from build123d import *

# Parameters (mm, degrees)
F0_W     = 115
F0_H     = 75
F1_DEPTH = 70
F2_W     = 60
F2_H     = 25
F3_DEPTH = 70
F4_W     = 10
F4_H     = 30
F5_DEPTH = 75
F6_W     = 30
F6_H     = 5
F6_W_2   = 15
F6_H_2   = 20
F7_DEPTH = 50
F8_W     = 25
F8_H     = 20
F9_DEPTH = 75


with BuildPart() as f1:
    # F0 (on Front) → F1 (new body)
    with BuildSketch(Plane.XZ):
        with Locations((57.5, 37.5)):
            Rectangle(F0_W, F0_H)
    extrude(amount=F1_DEPTH)

    # F2 (on face) → F3 (cut)
    with BuildSketch(Plane.XZ.offset(70)):
        with Locations((55, 62.5)):
            Rectangle(F2_W, F2_H)
    extrude(amount=-F3_DEPTH, mode=Mode.SUBTRACT)

    # F4 (on face) → F5 (cut)
    with BuildSketch(Plane.XY.offset(75)):
        with Locations((90, -55)):
            Rectangle(F4_W, F4_H)
    extrude(amount=-F5_DEPTH, mode=Mode.SUBTRACT)

    # F6 (on face) → F7 (cut)
    with BuildSketch(Plane.XY.offset(50)):
        Polygon((85, -70), (85, -40), (70, -40), (40, -40), (40, -50), (40, -70), align=None)
        with Locations((55, -37.5)):
            Rectangle(F6_W, F6_H)
        with Locations((32.5, -60)):
            Rectangle(F6_W_2, F6_H_2)
    extrude(amount=-F7_DEPTH, mode=Mode.SUBTRACT)

    # F8 (on face) → F9 (cut)
    with BuildSketch(Plane.XY.offset(75)):
        with Locations((12.5, -60)):
            Rectangle(F8_W, F8_H)
    extrude(amount=-F9_DEPTH, mode=Mode.SUBTRACT)


solid = f1.part
Design review of the part built by this model. Coordinates are the model's own, in mm. A direction names the side the tool comes from. Coordinates: 2 decimals unless noted, no trailing zeros. Order: outer loops, then holes, each group sorted by start corner. A loop starts at its lowest first (then second) coordinate and runs counter-clockwise, first axis right, second up. Notation, with made-up numbers: (-14, 85.25) -> (17, 85.25) arc R20 cw to (17, 117.25) -> close; hole circle Ø7 at (-10.5, 72.25). An arc over 180 degrees is marked (long way). Use one line per item in the form item = value. Start each with the question number.
(1) The part is to be moulded in two halves that separate along X. For faces 4 (the flat face through (0, -25, 37)), 5 (the flat face through (85, -20, 62)), 6 (the flat face through (115, -35, 37)), 7 (the flat face through (103, -35, 75)), say which applies: +X half, -X half, draft (parallel to the pull), parting line (faces both ways), or undercut.
(2) For faces 1 (the flat face through (20, -50, 38)), 2 (the flat face through (70, -38, 25)), 3 (the flat face through (25, -25, 63)), list the 3-axis set-ups (+Z, -Z, +X, -X, +Y, -Y) from which the entire face can be reached by the end or side of a thin tool; tool diameter is ignored.
(3) Add section D-D on x = 75.5. State the section outline as (y, z) points.
(4) Insertion check: pin 1 (3 mm diameter, centred on x = 63, y = -27, fed in from +Z); pin 2 (2 mm diameter, centred on x = 91, z = 23, fed in from -Y). Each pin has a flat end and moves straight along its axis. Give the tip position at first contact, or say it passes through.
(5) For probe 1 along X at (y, z) = (-36, 4.5); probe 2 along X at (y, z) = (-11, 64); probe 3 along Y at (x, z) = (51.5, 28), list the stretches that pass through material, from the lowest coordinate up.
(6) Add section A-A on z = 65. State the section outline as (x, y) points, plus the area to 3 significant figures.
(7) Add section B-B on z = 20. State the section outline as (x, y) points.
(8) Add section C-C on y = -7.5. State the section outline as (x, z) points.
Answer block:
q1.face_4 = -X half
q1.face_5 = undercut
q1.face_6 = +X half
q1.face_7 = draft
q2.face_1 = +Z, -Z, -X, -Y
q2.face_2 = +Z, -Z, -Y
q2.face_3 = +Z, +Y, -Y
q3.outline = (-40, 0) -> (0, 0) -> (0, 50) -> (-40, 50) -> close
q4.pin_1 = 50
q4.pin_2 = -40
q5.probe_1 = 0 to 40, 70 to 115
q5.probe_2 = 0 to 25, 85 to 115
q5.probe_3 = -35 to 0
q6.outline = (0, -50) -> (25, -50) -> (25, 0) -> (0, 0) -> close; (85, -40) -> (95, -40) -> (95, -70) -> (115, -70) -> (115, 0) -> (85, 0) -> close
q6.area = 3,050 mm²
q7.outline = (0, -50) -> (40, -50) -> (40, -35) -> (70, -35) -> (70, -40) -> (95, -40) -> (95, -70) -> (115, -70) -> (115, 0) -> (0, 0) -> close
q8.outline = (0, 0) -> (115, 0) -> (115, 75) -> (85, 75) -> (85, 50) -> (25, 50) -> (25, 75) -> (0, 75) -> close
